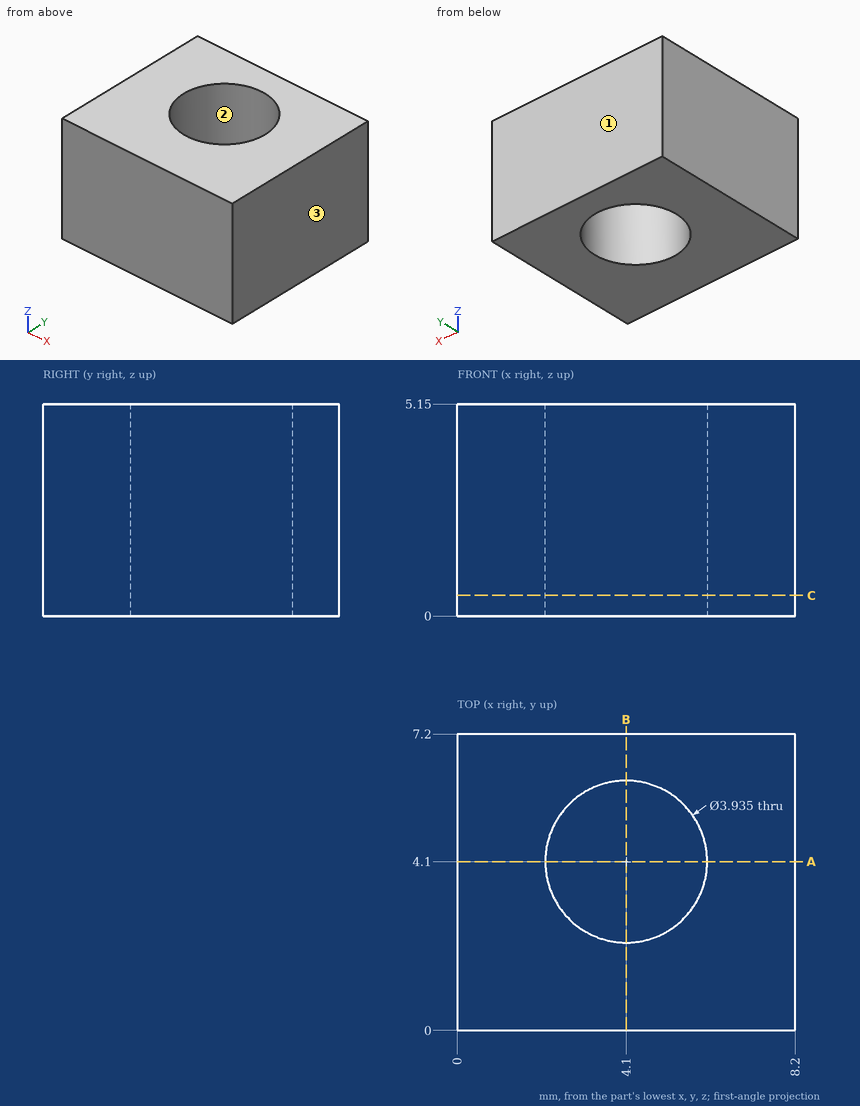
For this review, use the dimensioned drawing (mm, ordinates from the lowest corner) and the shaded views. Coordinates: 2 decimals unless noted, no trailing zeros. Order: outer loops, then holes, each group sorted by start corner. A loop starts at its lowest first (then second) coordinate and runs counter-clockwise, first axis right, second up. Notation, with made-up numbers: (14, 60) -> (61, 60) arc R26 cw to (61, 88) -> close; hole circle Ø2 at (65.5, 69.5). An arc over 180 degrees is marked (long way). One line per item, written item: value. Start each with the question number.
Q1. Mouldability with a two-part tool opening along Y and no side actions: class the marked faces 1, 2 and 3 as pulls with the +Y half, pulls with the -Y half, needs draft (parallel to the pull), parting line crosses it, or undercut.
Q2. Take a section at B-B, the plane x = 4.1. State the section outline as (y, z) points, then the cut area to 3 significant figures.
Q3. For probe 1 along Y at (x, z) = (4.1, 3.7); probe 2 along X at (y, z) = (5.75, 4.8); probe 3 along X at (y, z) = (3.5, 4.45), list the stretches that pass through material, from the lowest coordinate up.
Q4. Take a section at A-A, the plane y = 4.1. State the section outline as (x, z) points.
Q5. Take a section at C-C, the plane z = 0.5. State the section outline as (x, y) points (1 decimal), then the cut area to 3 significant figures.
Values follow:
1. face 1: pulls with the +Y half
1. face 2: undercut
1. face 3: needs draft
2. outline: (0, 0) -> (2.13, 0) -> (2.13, 5.15) -> (0, 5.15) -> close; (6.07, 0) -> (7.2, 0) -> (7.2, 5.15) -> (6.07, 5.15) -> close
2. area: 16.8 mm2
3. probe 1: y = 0 to 2.13, 6.07 to 7.2
3. probe 2: x = 0 to 3.03, 5.17 to 8.2
3. probe 3: x = 0 to 2.23, 5.97 to 8.2
4. outline: (0, 0) -> (2.13, 0) -> (2.13, 5.15) -> (0, 5.15) -> close; (6.07, 0) -> (8.2, 0) -> (8.2, 5.15) -> (6.07, 5.15) -> close
5. outline: (0, 0) -> (8.2, 0) -> (8.2, 7.2) -> (0, 7.2) -> close; hole circle Ø3.9 at (4.1, 4.1)
5. area: 46.9 mm2
